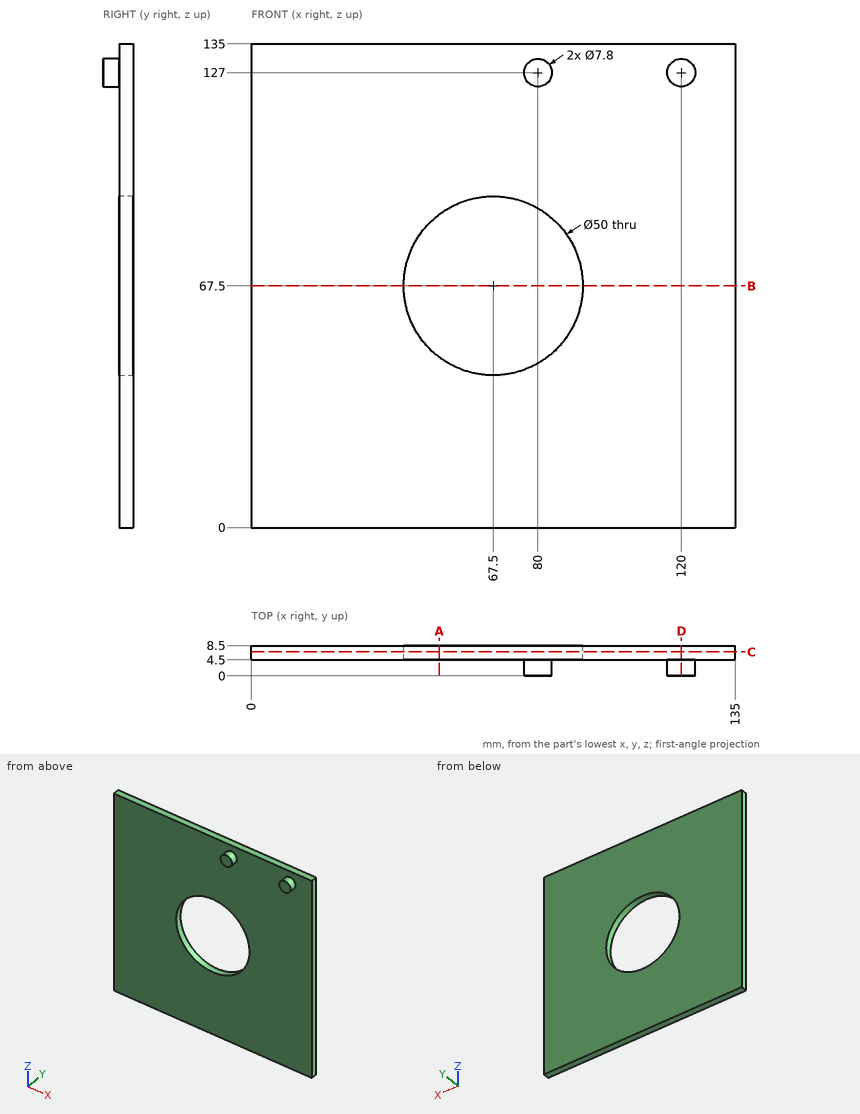
Job drawing, mm, ordinate dimensions from the low corner. One solid piece. Give positions to 0.01 mm unless a question says otherwise; leave off trailing zeros. Loops run counter-clockwise (first coordinate to the right, second up) from the corner with the lowest first, then second, coordinate; pieces in that order, holes last. Notation, with made-up numbers: M -36.5,87 L 13.5,87 A22 ccw 13.5,97 Z; hole C 36.5,-9 d4. An arc over 180 degrees is marked long. Return JSON: item names as keys, results as strings.
1) Drill centre lines: line 1 (X direction, y = 7.15, z = 67.5); line 2 (Y direction, x = 39.5, z = 84); line 3 (X direction, y = 6, z = 65). Where is each one in solid material? Low to high.
Calculated:
{"line 1": "x = 0 to 42.5, 92.5 to 135", "line 2": "y = 4.5 to 8.5", "line 3": "x = 0 to 42.63, 92.37 to 135"}
2) Saw through at C-C, the plane y = 6.75. List the corners of the cut face in (x, z).
Calculated:
{"outline": "M 0,0 L 135,0 L 135,135 L 0,135 Z; hole C 67.5,67.5 d50"}
3) Saw through at B-B, the plane z = 67.5. List the corners of the cut face in (x, y), then the cut area to 3 significant figures.
Calculated:
{"outline": "M 0,4.5 L 42.5,4.5 L 42.5,8.5 L 0,8.5 Z; M 92.5,4.5 L 135,4.5 L 135,8.5 L 92.5,8.5 Z", "area": "340 mm2"}
4) Flat gauge pins, fed straight in: pin 1 Ø3 at (x, y) = (48.5, 4.5) entering from -Z; pin 2 Ø12 at (x, z) = (20.5, 77) entering from -Y. Where does each tip first touch, or does it go through?
Calculated:
{"pin 1": "stops at z = 0", "pin 2": "stops at y = 4.5"}
5) Saw through at A-A, the plane x = 52.5. List the corners of the cut face in (y, z).
Calculated:
{"outline": "M 4.5,0 L 8.5,0 L 8.5,47.5 L 4.5,47.5 Z; M 4.5,87.5 L 8.5,87.5 L 8.5,135 L 4.5,135 Z"}
6) Saw through at D-D, the plane x = 120. List the corners of the cut face in (y, z), then the cut area to 3 significant figures.
Calculated:
{"outline": "M 0,123.1 L 4.5,123.1 L 4.5,0 L 8.5,0 L 8.5,135 L 4.5,135 L 4.5,130.9 L 0,130.9 Z", "area": "575 mm2"}
